The listing builds one solid part. Answer for the finished solid, in the listing's coordinates (mm). Coordinates: 2 decimals unless noted, no trailing zeros. Write each loop counter-clockwise with the first axis right and the second up, starting at its lowest first coordinate (ties: lowest second). Pieces come first, ordered by that corner, then holes. Notation, with made-up numbers: M 72.25,-4 L 89.25,-4 A24 cw 89.25,9 Z; hole C 83,40 d11. An arc over 180 degrees is marked long. Answer as CSV lines item,"result".
Autodesk Inventor part; units mm, degrees
ref_plane "YZ Plane" through (0, 0, 0) normal (1, 0, 0) x (0, 1, 0)
ref_plane "XZ Plane" through (0, 0, 0) normal (0, 1, 0) x (-1, 0, 0)
ref_plane "XY Plane" through (0, 0, 0) normal (0, 0, 1) x (1, 0, 0)
sketch "Sketch1" plane through (0, 0, 0) normal (0, 1, 0) x (-1, 0, 0)
  line L0 (-35, 35) -> (35, 35)
  line L1 (35, 35) -> (35, -35)
  line L2 (35, -35) -> (-35, -35)
  line L3 (-35, -35) -> (-35, 35)
  line L4 (-35, 35) -> (35, -35) construction
  line L5 (35, 35) -> (-35, -35) construction
  line L6 (-22.5, 22.5) -> (22.5, 22.5) construction
  line L7 (22.5, 22.5) -> (22.5, -22.5) construction
  line L8 (22.5, -22.5) -> (-22.5, -22.5) construction
  line L9 (-22.5, -22.5) -> (-22.5, 22.5) construction
  line L10 (-22.5, 22.5) -> (22.5, -22.5) construction
  line L11 (22.5, 22.5) -> (-22.5, -22.5) construction
  circle A0 centre (0, 0) radius 7
  line L12 (17.5, 22.5) -> (-17.5, 22.5) construction
  line L13 (-17.5, 22.5) -> (-17.5, -22.5) construction
  line L14 (-17.5, -22.5) -> (17.5, -22.5) construction
  line L15 (17.5, -22.5) -> (17.5, 22.5) construction
  line L16 (49, 0) -> (-49, 0) construction
  line L17 (0, -49) -> (0, 49) construction
  dimension "d0" = 70
  dimension "d1" = 45
  dimension "d2" = 14
  dimension "d19" = 70
  dimension "d20" = 35
  dimension "d21" = 45
  dimension "d25" = 12.5
  dimension "d26" = 17.5
extrude "Extrusion1" add sketch "Sketch1" against normal blind 12
hole "Hole1" at (-22.5, 0, 22.5) at (22.5, 0, 22.5) at (-17.5, 0, -22.5) at (17.5, 0, -22.5) direction (0, -1, 0) diameter 8.376 end through all
chamfer "Chamfer1" distance 1 angle 45 8 edges at (17.5, 0, -26.688) (-17.5, 0, -26.688) (22.5, 0, 18.312) (-22.5, 0, 18.312) (17.5, -12, -26.688) (-17.5, -12, -26.688) (22.5, -12, 18.312) (-22.5, -12, 18.312)
chamfer "Chamfer2" distance 0.5 angle 45 2 edges at (7, 0, 0) (7, -12, 0)
chamfer "Chamfer3" distance 1 angle 45 4 edges at (-35, -6, 35) (-35, -6, -35) (35, -6, -35) (35, -6, 35)
properties part number "AP1-001"
Q1. The mould has two halves that part along Z. Classify faces 1 (the cylindrical face through (14.67, -6.07, -25.587)), 2 (the flat face through (0, -6, -35)), 3 (the flat face through (0, -6, 35)), 4 (the flat face through (0, -12, 8)): pulls with the +Z half, pulls with the -Z half, needs draft (parallel to the pull), parting line crosses it, or undercut.
Output:
face 1,"undercut"
face 2,"pulls with the -Z half"
face 3,"pulls with the +Z half"
face 4,"needs draft"
Q2. Straight lines are drawn through the part: line 1 (X direction, y = -3.75, z = -22.5); line 2 (X direction, y = -7, z = 22.5); line 3 (Z direction, x = 22.5, y = -3.25). For each, find the intervals that lie inside material, in ascending order.
Output:
line 1,"-35 to -21.69, -13.31 to 13.31, 21.69 to 35"
line 2,"-35 to -26.69, -18.31 to 18.31, 26.69 to 35"
line 3,"-35 to 18.31, 26.69 to 35"
Q3. Find section D-D (z = 22.5). Give the vertices of the cut face in (x, y), and give its area (3 significant figures).
Output:
outline,"M -35,-12 L -27.69,-12 L -26.69,-11 L -26.69,-1 L -27.69,0 L -35,0 Z; M -18.31,-11 L -17.31,-12 L 17.31,-12 L 18.31,-11 L 18.31,-1 L 17.31,0 L -17.31,0 L -18.31,-1 Z; M 26.69,-11 L 27.69,-12 L 35,-12 L 35,0 L 27.69,0 L 26.69,-1 Z"
area,"635 mm2"
Q4. A flat-ended cylindrical pin translates along its axis: pin 1 Ø18 at (x, z) = (0, 0) entering from +Y. Find the tip coordinate at first contact, or state that the pin passes through.
Output:
pin 1,"y = 0"
Q5. Find section C-C (y = -7.25). Give the vertices of the cut face in (x, z).
Output:
outline,"M -35,-34 L -34,-35 L 34,-35 L 35,-34 L 35,34 L 34,35 L -34,35 L -35,34 Z; hole C -22.5,22.5 d8.38; hole C -17.5,-22.5 d8.38; hole C 0,0 d14; hole C 17.5,-22.5 d8.38; hole C 22.5,22.5 d8.38"
Q6. Find section A-A (z = 0). Give the vertices of the cut face in (x, y).
Output:
outline,"M -35,-12 L -7.5,-12 L -7,-11.5 L -7,-0.5 L -7.5,0 L -35,0 Z; M 7,-11.5 L 7.5,-12 L 35,-12 L 35,0 L 7.5,0 L 7,-0.5 Z"
Q7. Find section B-B (x = 0). Give the vertices of the cut face in (y, z), and give its area (4 significant figures).
Output:
outline,"M -12,-35 L 0,-35 L 0,-7.5 L -0.5,-7 L -11.5,-7 L -12,-7.5 Z; M -12,7.5 L -11.5,7 L -0.5,7 L 0,7.5 L 0,35 L -12,35 Z"
area,"671.5 mm2"
